The listing builds one solid part. Answer for the finished solid, in the listing's coordinates (mm). Face numbers are marked on the shaded views. Give positions to 0.01 mm unless a question says otherwise; leave off trailing zeros. Order: outer loops, then holes, each group sorted by start corner. A loop starts at its lowest first (then second) coordinate and runs counter-clockwise, first axis right, second up. Notation, with made-up numbers: (34.5, -16) - (38.5, -16) arc R14 cw to (38.5, 7) - close; hole circle Ø2 at (-18.5, 48). An arc over 180 degrees is marked (long way). Answer as a JSON object with one key per item and string values. Group by question number.
Q1. Consider line 1 (X direction, y = 37.5, z = 0); line 2 (X direction, y = 111, z = -60.5); line 3 (Z direction, x = -14, y = 190). Determine where each line is inside the solid, lowest interval first.
Q2. A cutting plane is placed at A-A, the plane z = 0. Give the vertices of the cut face in (x, y), and give its area (3 significant figures).
Q3. The mould has two halves that part along X. Classify the marked faces 1 and 2: released by +X, released by -X, zero draft, split by the parting line, or undercut.
Q4. Given pin 1 (2 mm diameter, centred on y = 204, z = 12.5, fed in from -X); pin 2 (3 mm diameter, centred on x = 13.5, y = 248.5, fed in from -Z); pin 3 (6 mm diameter, centred on x = -6, y = 273.5, fed in from +Z); pin 4 (4.5 mm diameter, centred on x = 0, y = 4.76, fed in from -Z), each flat-ended and moving along its own axis, determine where each tip first touches the part or whether it passes through.
Q5. A cutting plane is placed at B-B, the plane x = 54. Give the vertices of the cut face in (y, z), and give its area (3 significant figures).
Q6. A cutting plane is placed at C-C, the plane y = 244. Give the vertices of the cut face in (x, z), and give its area (3 significant figures).
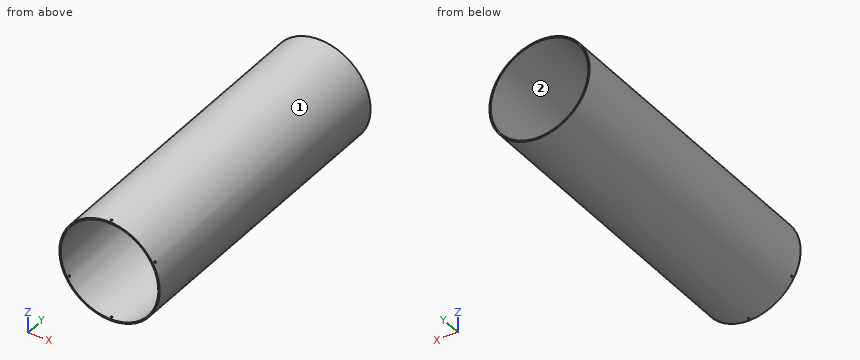
from build123d import *

# Parameters (mm, degrees)
SKETCH1_R           = 78.359
SKETCH1_R_2         = 76.2
BOSS_EXTRUDE1_DEPTH = 482.6
SKETCH2_R           = 1.35255
CUT_EXTRUDE1_DEPTH  = 496.159596254
CIRPATTERN1_COUNT   = 6


with BuildPart() as part:
    # Sketch1 → Boss-Extrude1 (new body)
    with BuildSketch(Plane(origin=(0, 0, 0), x_dir=(1, 0, 0), z_dir=(0, 1, 0))):
        with Locations(Location((0, 0, 0), (0, 0, 90))):
            Circle(SKETCH1_R)
        with Locations(Location((0, 0, 0), (0, 0, 90))):
            Circle(SKETCH1_R_2, mode=Mode.SUBTRACT)
    extrude(amount=BOSS_EXTRUDE1_DEPTH)

    # Sketch2 → Cut-Extrude1 (cut, through all)
    with BuildSketch(Plane.XY):
        with Locations(Location((0, 4.7625, 0), (0, 0, 90))):
            Circle(SKETCH2_R)
    cut_extrude1 = extrude(amount=-CUT_EXTRUDE1_DEPTH, mode=Mode.SUBTRACT)

    # CirPattern1: Cut-Extrude1 ×6 about axis
    cirpattern1_axis = Axis((0, 482.6, 0), (0, -1, 0))
    for i in range(1, CIRPATTERN1_COUNT):
        add(cut_extrude1.rotate(cirpattern1_axis, i * 360 / CIRPATTERN1_COUNT), mode=Mode.SUBTRACT)


solid = part.part
Reply:
{
 "1": {"line 1": "x = -78.36 to -76.2, 76.2 to 78.36", "line 2": "x = -49.8 to -46.33, 46.33 to 49.8", "line 3": "z = -77.1 to -74.9, 74.9 to 77.1"},
 "2": {"outline": "(-78.36, 0) - (-76.2, 0) - (-76.2, 482.6) - (-78.36, 482.6) - close; (76.2, 0) - (78.36, 0) - (78.36, 482.6) - (76.2, 482.6) - close", "area": "2,080 mm^2"},
 "3": {"face 1": "split by the parting line", "face 2": "undercut"},
 "4": {"pin 1": "stops at x = -77.51", "pin 2": "stops at z = -77.43", "pin 3": "stops at z = 78.3", "pin 4": "stops at z = -78.36"},
 "5": {"outline": "(0, -56.78) - (482.6, -56.78) - (482.6, -53.76) - (0, -53.76) - close; (0, 53.76) - (482.6, 53.76) - (482.6, 56.78) - (0, 56.78) - close", "area": "2,910 mm^2"},
 "6": {"outline": "circle Ø156.72 at (0, 0); hole circle Ø152.4 at (0, 0)", "area": "1,050 mm^2"}
}
